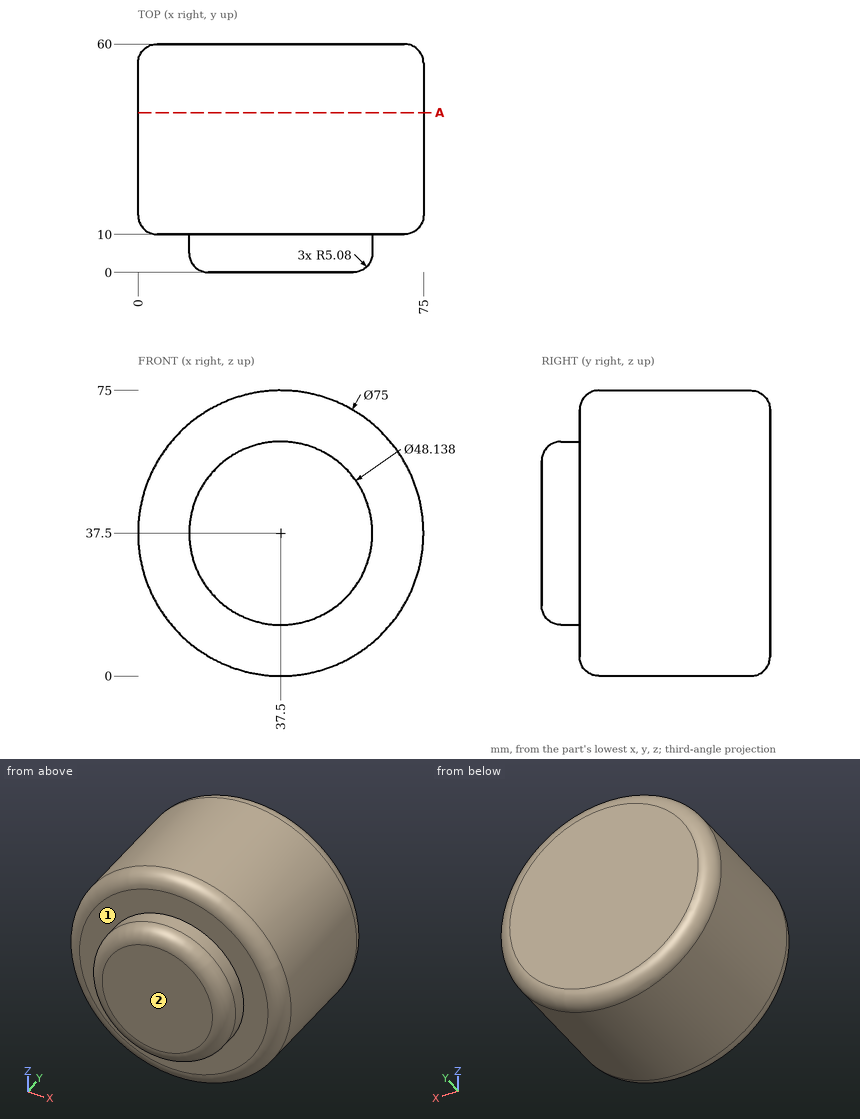
Source: three-view drawing plus pictorial views. Frame: mm from the lowest corner of the part. A direction names the side the tool comes from. Coordinates: 2 decimals unless noted, no trailing zeros. Loops run counter-clockwise (first coordinate to the right, second up) from the corner with the lowest first, then second, coordinate; pieces in that order, holes last. Notation, with made-up numbers: (84, 22.25) -> (125, 22.25) arc R28 cw to (125, 59.25) -> close; hole circle Ø2 at (70, -23.5). An arc over 180 degrees is marked (long way). Answer in a Markdown table with one row per item. Add a question column.
Q1. Reachability of the marked faces 1 and 2 from +Z, -Z, +X, -X, +Y, -Y: full face, straight path, thin tool, end or side. Return the list, or none.
Q2. Ray query, line 1 along Y through (x, z) = (53.5, 65); line 2 along X through (y, z) = (50, 65.5) (1 decimal); line 3 along X through (y, z) = (15, 11). Return the intervals inside material, ascending.
Q3. Contact query for flat-ended pins moving along their axis: pin 1 Ø1.5 at (y, z) = (23.5, 54.5) entering from -X; pin 2 Ø3 at (y, z) = (16.5, 16.5) entering from +X; pin 3 Ø5 at (x, y) = (64.5, 18.5) entering from -Z. Output: stop coordinate, or through.
Q4. Section A-A on y = 42. Return the cut outline in (x, z).
Computed values:
| question | item | result |
|---|---|---|
| 1 | face 1 | -Y |
| 1 | face 2 | +Z, -Z, +X, -X, -Y |
| 2 | line 1 | y = 10 to 60 |
| 2 | line 2 | x = 12.6 to 62.4 |
| 2 | line 3 | x = 10.97 to 64.03 |
| 3 | pin 1 | stops at x = 3.7 |
| 3 | pin 2 | stops at x = 69.53 |
| 3 | pin 3 | stops at z = 9.11 |
| 4 | outline | circle Ø75 at (37.5, 37.5) |
